```python
from build123d import *

# Parameters (mm, degrees)
SKETCH1_R                    = 21
BOSS_EXTRUDE1_DEPTH          = 24
BOSS_EXTRUDE1_DEPTH_BACK     = 24
SKETCH3_R                    = 7
CUT_EXTRUDE1_DEPTH           = 24
CUT_EXTRUDE1_TAPER           = -15
CUT_EXTRUDE1_OTHER_WAY_DEPTH = 24
SKETCH4_R                    = 21
BOSS_EXTRUDE2_DEPTH          = 10
SKETCH5_R                    = 7
CUT_EXTRUDE2_DEPTH           = 10
CUT_EXTRUDE2_TAPER           = -45


with BuildPart() as part:
    # Sketch1 → Boss-Extrude1 (new body, two sides)
    with BuildSketch(Plane(origin=(0, 0, 0), x_dir=(1, 0, 0), z_dir=(0, 1, 0))) as boss_extrude1_sk:
        Circle(SKETCH1_R)
    extrude(amount=BOSS_EXTRUDE1_DEPTH)
    extrude(boss_extrude1_sk.sketch, amount=-BOSS_EXTRUDE1_DEPTH_BACK)

    # Sketch3 → Cut-Extrude1 (cut)
    with BuildSketch(Plane(origin=(0, 0, 0), x_dir=(1, 0, 0), z_dir=(0, 1, 0))):
        Circle(SKETCH3_R)
    extrude(amount=-CUT_EXTRUDE1_DEPTH, taper=CUT_EXTRUDE1_TAPER, mode=Mode.SUBTRACT)

    # Sketch3 → Cut-Extrude1 other way (cut)
    with BuildSketch(Plane(origin=(0, 0, 0), x_dir=(1, 0, 0), z_dir=(0, 1, 0))):
        Circle(SKETCH3_R)
    extrude(amount=CUT_EXTRUDE1_OTHER_WAY_DEPTH, mode=Mode.SUBTRACT)

    # Sketch4 → Boss-Extrude2 (add)
    with BuildSketch(Plane(origin=(0, 24, 0), x_dir=(1, 0, 0), z_dir=(0, 1, 0))):
        Circle(SKETCH4_R)
    extrude(amount=BOSS_EXTRUDE2_DEPTH)

    # Sketch5 → Cut-Extrude2 (cut)
    with BuildSketch(Plane.XZ.offset(-24)):
        Circle(SKETCH5_R)
    extrude(amount=-CUT_EXTRUDE2_DEPTH, taper=CUT_EXTRUDE2_TAPER, mode=Mode.SUBTRACT)


solid = part.part
```
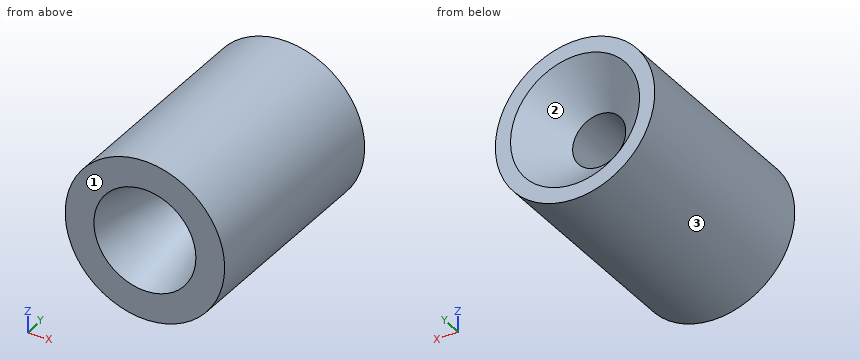
The model under review builds one solid part; all positions refer to its coordinate system, in mm. Face numbers are marked on the shaded views. Coordinates: 2 decimals unless noted, no trailing zeros. Write each loop counter-clockwise with the first axis right and the second up, starting at its lowest first coordinate (ties: lowest second). Pieces come first, ordered by that corner, then holes.
1) To check wall thickness, follow probe 1 along Z at (x, y) = (0, 7.5); probe 2 along Z at (x, y) = (-6, -9). State the ranges of each line that lie inside material, in increasing order.
2) The part is to be moulded in two halves that separate along Z. For the marked faces 1, 2 and 3, say which applies: pulls with the +Z half, pulls with the -Z half, needs draft (parallel to the pull), parting line crosses it, or undercut.
3) We need section C-C on y = 8. State the section outline as (x, z) points.
4) We need section A-A on x = 0. State the section outline as (y, z) points.
5) Clearance check with flat-ended pins moving along their axes: pin 1 Ø6 at (y, z) = (-8, -11) entering from +X; pin 2 Ø3 at (x, y) = (-15, 11) entering from -Z; pin 3 Ø2 at (y, z) = (-11, 5) entering from -X. State where each tip first meets the part, or that it passes through.
6) We need section B-B on y = 25. State the section outline as (x, z) points.
Answer list:
1. probe 1: z = -21 to -7, 7 to 21
1. probe 2: z = -20.12 to -7.25, 7.25 to 20.12
2. face 1: needs draft
2. face 2: undercut
2. face 3: parting line crosses it
3. outline: circle Ø42 at (0, 0); hole circle Ø14 at (0, 0)
4. outline: (-24, -21) - (34, -21) - (34, -17) - (24, -7) - (0, -7) - (-24, -13.43) - close; (-24, 13.43) - (0, 7) - (24, 7) - (34, 17) - (34, 21) - (-24, 21) - close
5. pin 1: stops at x = 19.42
5. pin 2: stops at z = -16.09
5. pin 3: stops at x = -20.62
6. outline: circle Ø42 at (0, 0); hole circle Ø16 at (0, 0)
